For this review, take the finished solid that the model builds, in its own axes (mm). A direction names the side the tool comes from. Give positions to 0.01 mm unless a question says otherwise; leave off trailing zeros. Order: outer loops, then holes, each group sorted by start corner. A loop starts at its lowest first (then second) coordinate and runs counter-clockwise, first axis right, second up. Notation, with made-up numbers: (4, 69) -> (11, 69) arc R20 ccw to (11, 87) -> close; hole circle Ø1 at (88, 60). An arc over 180 degrees is marked (long way). Return JSON: item names as keys, results as strings. Group by question number.
1) To check wall thickness, follow line 1 along X through (y, z) = (23, -7.5); line 2 along Z through (x, y) = (64, 23); line 3 along Z through (x, y) = (10, 0.25). State the ranges of each line that lie inside material, in increasing order.
2) Insertion check: P1, Ø1.6, axis at x = -39.5, y = 17, coming from the +Z side; P2, Ø2, axis at x = 14.5, z = 20, coming from the +Y side; P3, Ø2.5, axis at x = 34, z = 31, coming from the +Y side; P4, Ø4.5, axis at x = 67.5, z = -47.5, coming from the -Y side. Each pin has a flat end and moves straight along its axis. Give the tip position at first contact, or say it passes through.
3) Add section B-B (y = 12). Give the boundary of the cut face in (x, z), then the cut area to 3 significant figures.
4) Add section A-A (y = 20.5). Give the boundary of the cut face in (x, z).
5) The part is to be moulded in two halves that separate along Z. For faces 5 (the face through (0, 2, 47)), 6 (the face through (29, 9, -34.3)), 7 (the face through (-67, 3, -55)), say which applies: released by +Z, released by -Z, zero draft, split by the parting line, or undercut.
6) Add section D-D (x = 67.5). Give the boundary of the cut face in (y, z), then the cut area to 3 significant figures.
7) For faces 1 (the face through (12, 9, -34.118)), 2 (the face through (57.5, 2, -47)), 3 (the face through (-70, 5, -44)), 4 (the face through (12, 5, 44)), list the 3-axis set-ups (+Z, -Z, +X, -X, +Y, -Y) from which the entire face can be reached by the end or side of a thin tool; tool diameter is ignored.
8) Add section C-C (z = -47.5). Give the boundary of the cut face in (x, y), then the cut area to 3 significant figures.
from build123d import *

# Parameters (mm, degrees)
SKETCH1_W            = 155
SKETCH1_H            = 80
BOSS_EXTRUDE1_DEPTH  = 2
SKETCH3_R            = 1.45
BOSS_EXTRUDE2_DEPTH  = 5
SKETCH4_W            = 5
SKETCH4_H            = 3
BOSS_EXTRUDE3_DEPTH  = 14
SKETCH5_W            = 5
SKETCH5_H            = 3
BOSS_EXTRUDE4_DEPTH  = 14
SKETCH6_W            = 10
SKETCH6_H            = 3
BOSS_EXTRUDE5_DEPTH  = 14
SKETCH7_W            = 2
SKETCH7_H            = 3
BOSS_EXTRUDE6_DEPTH  = 21
SKETCH8_W            = 155
SKETCH8_H            = 1.5
BOSS_EXTRUDE7_DEPTH  = 35
SKETCH9_W            = 155
SKETCH9_H            = 1.5
BOSS_EXTRUDE8_DEPTH  = 35
SKETCH10_W           = 1.5
SKETCH10_H           = 77
BOSS_EXTRUDE9_DEPTH  = 35
SKETCH11_W           = 1.5
SKETCH11_H           = 77
BOSS_EXTRUDE10_DEPTH = 35
SKETCH12_W           = 4
SKETCH12_H           = 8
CUT_EXTRUDE1_DEPTH   = 5
SKETCH13_W           = 4
SKETCH13_H           = 8
CUT_EXTRUDE2_DEPTH   = 5
SKETCH14_W           = 20
SKETCH14_H           = 5
BOSS_EXTRUDE11_DEPTH = 15
SKETCH15_W           = 20
SKETCH15_H           = 5
BOSS_EXTRUDE12_DEPTH = 15
SKETCH16_R           = 1.95
CUT_EXTRUDE3_DEPTH   = 5
SKETCH17_R           = 3.5
CUT_EXTRUDE4_DEPTH   = 10
CUT_EXTRUDE4_DRAFT   = -18
SKETCH18_R           = 1.95
CUT_EXTRUDE5_DEPTH   = 10
SKETCH19_R           = 3.5
CUT_EXTRUDE6_DEPTH   = 10
CUT_EXTRUDE6_DRAFT   = -18
SKETCH20_R           = 1.95
CUT_EXTRUDE7_DEPTH   = 10
SKETCH21_R           = 3.5
CUT_EXTRUDE8_DEPTH   = 10
CUT_EXTRUDE8_DRAFT   = -18
SKETCH22_R           = 1.45
CUT_EXTRUDE9_DEPTH   = 200
SKETCH23_R           = 1.45
CUT_EXTRUDE10_DEPTH  = 200


with BuildPart() as part:
    # Sketch1 → Boss-Extrude1 (new body)
    with BuildSketch(Plane(origin=(0, 0, 0), x_dir=(1, 0, 0), z_dir=(0, 1, 0))):
        Rectangle(SKETCH1_W, SKETCH1_H)
    extrude(amount=BOSS_EXTRUDE1_DEPTH)

    # Sketch3 → Boss-Extrude2 (add)
    with BuildSketch(Plane(origin=(0, 2, 0), x_dir=(1, 0, 0), z_dir=(0, 1, 0))):
        with Locations(Location((-20.3, -24.15, 0), (0, 0, 270))):
            Circle(SKETCH3_R)
        with Locations(Location((-19, 24.05, 0), (0, 0, 270))):
            Circle(SKETCH3_R)
        with Locations(Location((31.8, 8.85, 0), (0, 0, 270))):
            Circle(SKETCH3_R)
        with Locations(Location((31.8, -19.05, 0), (0, 0, 270))):
            Circle(SKETCH3_R)
    extrude(amount=BOSS_EXTRUDE2_DEPTH)

    # Sketch4 → Boss-Extrude3 (add)
    with BuildSketch(Plane(origin=(0, 2, 0), x_dir=(1, 0, 0), z_dir=(0, 1, 0))):
        with Locations((29.3, 32.8)):
            Rectangle(SKETCH4_W, SKETCH4_H)
    extrude(amount=BOSS_EXTRUDE3_DEPTH)

    # Sketch5 → Boss-Extrude4 (add)
    with BuildSketch(Plane(origin=(0, 2, 0), x_dir=(1, 0, 0), z_dir=(0, 1, 0))):
        with Locations((12.287448128, 32.618143972)):
            Rectangle(SKETCH5_W, SKETCH5_H)
    extrude(amount=BOSS_EXTRUDE4_DEPTH)

    # Sketch6 → Boss-Extrude5 (add)
    with BuildSketch(Plane(origin=(0, 2, 0), x_dir=(1, 0, 0), z_dir=(0, 1, 0))):
        with Locations((31.8, -30.5)):
            Rectangle(SKETCH6_W, SKETCH6_H)
    extrude(amount=BOSS_EXTRUDE5_DEPTH)

    # Sketch7 → Boss-Extrude6 (add)
    with BuildSketch(Plane(origin=(0, 2, 0), x_dir=(1, 0, 0), z_dir=(0, 1, 0))):
        with Locations((-39.555823147, -25.65)):
            Rectangle(SKETCH7_W, SKETCH7_H)
    extrude(amount=BOSS_EXTRUDE6_DEPTH)

    # Sketch8 → Boss-Extrude7 (add)
    with BuildSketch(Plane(origin=(0, 2, 0), x_dir=(1, 0, 0), z_dir=(0, 1, 0))):
        with Locations((0, 39.25)):
            Rectangle(SKETCH8_W, SKETCH8_H)
    extrude(amount=BOSS_EXTRUDE7_DEPTH)

    # Sketch9 → Boss-Extrude8 (add)
    with BuildSketch(Plane(origin=(0, 2, 0), x_dir=(1, 0, 0), z_dir=(0, 1, 0))):
        with Locations((0, -39.25)):
            Rectangle(SKETCH9_W, SKETCH9_H)
    extrude(amount=BOSS_EXTRUDE8_DEPTH)

    # Sketch10 → Boss-Extrude9 (add)
    with BuildSketch(Plane(origin=(0, 2, 0), x_dir=(1, 0, 0), z_dir=(0, 1, 0))):
        with Locations((76.75, 0)):
            Rectangle(SKETCH10_W, SKETCH10_H)
    extrude(amount=BOSS_EXTRUDE9_DEPTH)

    # Sketch11 → Boss-Extrude10 (add)
    with BuildSketch(Plane(origin=(0, 2, 0), x_dir=(1, 0, 0), z_dir=(0, 1, 0))):
        with Locations((-76.75, 0)):
            Rectangle(SKETCH11_W, SKETCH11_H)
    extrude(amount=BOSS_EXTRUDE10_DEPTH)

    # Sketch12 → Cut-Extrude1 (cut)
    with BuildSketch(Plane.ZY.offset(77.5)):
        with Locations((0, 37)):
            Rectangle(SKETCH12_W, SKETCH12_H)
    extrude(amount=-CUT_EXTRUDE1_DEPTH, mode=Mode.SUBTRACT)

    # Sketch13 → Cut-Extrude2 (cut)
    with BuildSketch(Plane(origin=(77.5, 0, 0), x_dir=(0, 0, -1), z_dir=(1, 0, 0))):
        with Locations((0, 37)):
            Rectangle(SKETCH13_W, SKETCH13_H)
    extrude(amount=-CUT_EXTRUDE2_DEPTH, mode=Mode.SUBTRACT)

    # Sketch14 → Boss-Extrude11 (add)
    with BuildSketch(Plane(origin=(0, 0, -40), x_dir=(-1, 0, 0), z_dir=(0, 0, -1))):
        with Locations((-67.5, 2.5)):
            Rectangle(SKETCH14_W, SKETCH14_H)
        with Locations((67.5, 2.5)):
            Rectangle(SKETCH14_W, SKETCH14_H)
    extrude(amount=BOSS_EXTRUDE11_DEPTH)

    # Sketch15 → Boss-Extrude12 (add)
    with BuildSketch(Plane.XY.offset(40)):
        with Locations((10, 2.5)):
            Rectangle(SKETCH15_W, SKETCH15_H)
    extrude(amount=BOSS_EXTRUDE12_DEPTH)

    # Sketch16 → Cut-Extrude3 (cut)
    with BuildSketch(Plane(origin=(0, 5, 0), x_dir=(1, 0, 0), z_dir=(0, 1, 0))):
        with Locations(Location((67.5, 47.5, 0), (0, 0, 270))):
            Circle(SKETCH16_R)
    extrude(amount=-CUT_EXTRUDE3_DEPTH, mode=Mode.SUBTRACT)


with BuildPart() as cut_extrude4_tool:
    # Sketch17 → Cut-Extrude4 (with draft: the straight prism first)
    with BuildSketch(Plane(origin=(0, 5, 0), x_dir=(1, 0, 0), z_dir=(0, 1, 0))):
        with Locations((67.5, 47.5)):
            Circle(SKETCH17_R)
    extrude(amount=-CUT_EXTRUDE4_DEPTH)
    # Cut-Extrude4: the draft: its side faces are tilted about the plane it starts from
    cut_extrude4_sides = [cut_extrude4_tool.faces().sort_by_distance(p)[0] for p in [
        (64, 0, -47.5),
    ]]
    draft(cut_extrude4_sides, Plane(origin=(0, 5, 0), x_dir=(1, 0, 0), z_dir=(0, 1, 0)), CUT_EXTRUDE4_DRAFT)


with BuildPart() as part_1:
    add(part.part)

    # Cut-Extrude4: cut by cut_extrude4_tool
    add(cut_extrude4_tool.part, mode=Mode.SUBTRACT)

    # Sketch18 → Cut-Extrude5 (cut)
    with BuildSketch(Plane(origin=(0, 5, 0), x_dir=(1, 0, 0), z_dir=(0, 1, 0))):
        with Locations(Location((-67.5, 47.5, 0), (0, 0, 180))):
            Circle(SKETCH18_R)
    extrude(amount=-CUT_EXTRUDE5_DEPTH, mode=Mode.SUBTRACT)


with BuildPart() as cut_extrude6_tool:
    # Sketch19 → Cut-Extrude6 (with draft: the straight prism first)
    with BuildSketch(Plane(origin=(0, 5, 0), x_dir=(1, 0, 0), z_dir=(0, 1, 0))):
        with Locations((-67.5, 47.5)):
            Circle(SKETCH19_R)
    extrude(amount=-CUT_EXTRUDE6_DEPTH)
    # Cut-Extrude6: the draft: its side faces are tilted about the plane it starts from
    cut_extrude6_sides = [cut_extrude6_tool.faces().sort_by_distance(p)[0] for p in [
        (-71, 0, -47.5),
    ]]
    draft(cut_extrude6_sides, Plane(origin=(0, 5, 0), x_dir=(1, 0, 0), z_dir=(0, 1, 0)), CUT_EXTRUDE6_DRAFT)


with BuildPart() as part_2:
    add(part_1.part)

    # Cut-Extrude6: cut by cut_extrude6_tool
    add(cut_extrude6_tool.part, mode=Mode.SUBTRACT)

    # Sketch20 → Cut-Extrude7 (cut)
    with BuildSketch(Plane(origin=(0, 5, 0), x_dir=(1, 0, 0), z_dir=(0, 1, 0))):
        with Locations(Location((10, -47.5, 0), (0, 0, 270))):
            Circle(SKETCH20_R)
    extrude(amount=-CUT_EXTRUDE7_DEPTH, mode=Mode.SUBTRACT)


with BuildPart() as cut_extrude8_tool:
    # Sketch21 → Cut-Extrude8 (with draft: the straight prism first)
    with BuildSketch(Plane(origin=(0, 5, 0), x_dir=(1, 0, 0), z_dir=(0, 1, 0))):
        with Locations((10, -47.5)):
            Circle(SKETCH21_R)
    extrude(amount=-CUT_EXTRUDE8_DEPTH)
    # Cut-Extrude8: the draft: its side faces are tilted about the plane it starts from
    cut_extrude8_sides = [cut_extrude8_tool.faces().sort_by_distance(p)[0] for p in [
        (6.5, 0, 47.5),
    ]]
    draft(cut_extrude8_sides, Plane(origin=(0, 5, 0), x_dir=(1, 0, 0), z_dir=(0, 1, 0)), CUT_EXTRUDE8_DRAFT)


with BuildPart() as part_3:
    add(part_2.part)

    # Cut-Extrude8: cut by cut_extrude8_tool
    add(cut_extrude8_tool.part, mode=Mode.SUBTRACT)

    # Sketch22 → Cut-Extrude9 (cut)
    with BuildSketch(Plane(origin=(77.5, 0, 0), x_dir=(0, 0, -1), z_dir=(1, 0, 0))):
        with Locations((-34.5, 32)):
            Circle(SKETCH22_R)
    extrude(amount=-CUT_EXTRUDE9_DEPTH, mode=Mode.SUBTRACT)

    # Sketch23 → Cut-Extrude10 (cut)
    with BuildSketch(Plane(origin=(77.5, 0, 0), x_dir=(0, 0, -1), z_dir=(1, 0, 0))):
        with Locations((34.5, 32)):
            Circle(SKETCH23_R)
    extrude(amount=-CUT_EXTRUDE10_DEPTH, mode=Mode.SUBTRACT)


solid = part_3.part
Evaluation:
{
 "1": {"line 1": "-77.5 to -76, 76 to 77.5", "line 2": "-40 to -38.5, 38.5 to 40", "line 3": "-40 to 45.54, 49.46 to 55"},
 "2": {"P1": "z = 40", "P2": "y = 2", "P3": "y = 16", "P4": "y = 0"},
 "3": {"outline": "(-77.5, -40) -> (77.5, -40) -> (77.5, 40) -> (-77.5, 40) -> close; (-40.56, 24.15) -> (-38.56, 24.15) -> (-38.56, 27.15) -> (-40.56, 27.15) -> close; (9.79, -34.12) -> (14.79, -34.12) -> (14.79, -31.12) -> (9.79, -31.12) -> close; (26.8, -34.3) -> (31.8, -34.3) -> (31.8, -31.3) -> (26.8, -31.3) -> close; (26.8, 29) -> (36.8, 29) -> (36.8, 32) -> (26.8, 32) -> close; hole (-76, -38.5) -> (76, -38.5) -> (76, 38.5) -> (-76, 38.5) -> close", "area": "762 mm^2"},
 "4": {"outline": "(-77.5, -40) -> (77.5, -40) -> (77.5, 40) -> (-77.5, 40) -> close; (-40.56, 24.15) -> (-38.56, 24.15) -> (-38.56, 27.15) -> (-40.56, 27.15) -> close; hole (-76, -38.5) -> (76, -38.5) -> (76, 38.5) -> (-76, 38.5) -> close"},
 "5": {"face 5": "zero draft", "face 6": "undercut", "face 7": "released by -Z"},
 "6": {"outline": "(0, -55) -> (5, -55) -> (5, -51) -> (0.23, -49.45) -> (0, -49.45) -> close; (0, -45.55) -> (0.23, -45.55) -> (5, -44) -> (5, -40) -> (37, -40) -> (37, -38.5) -> (2, -38.5) -> (2, 38.5) -> (37, 38.5) -> (37, 40) -> (0, 40) -> close", "area": "313 mm^2"},
 "7": {"face 1": "+Y", "face 2": "-Z, +Y, -Y", "face 3": "-Z, +X, -X, +Y", "face 4": "+Z, +X, -X, +Y"},
 "8": {"outline": "(-77.5, 0) -> (-69.45, 0) -> (-69.45, 0.23) -> (-71, 5) -> (-77.5, 5) -> close; (-65.55, 0) -> (-57.5, 0) -> (-57.5, 5) -> (-64, 5) -> (-65.55, 0.23) -> close; (57.5, 0) -> (65.55, 0) -> (65.55, 0.23) -> (64, 5) -> (57.5, 5) -> close; (69.45, 0) -> (77.5, 0) -> (77.5, 5) -> (71, 5) -> (69.45, 0.23) -> close", "area": "146 mm^2"}
}
